Drawing for the job (mm, zero at the part's lowest x, y, z). A direction names the side the tool comes from. Round coordinates to 2 decimals unless told otherwise and drop trailing zeros. Loops run counter-clockwise (first coordinate to the right, second up) from the corner with the lowest first, then second, coordinate; pieces in that order, holes last. Notation, with made-up numbers: (-26.5, 26.25) -> (26.5, 26.25) arc R10 cw to (26.5, 41.25) -> close; hole circle Ø2 at (78.25, 80.25). An arc over 180 degrees is marked (long way). Put each result on its own line as item: value. Start each with the question number.
Item 1: Drill centre lines: probe 1 along Y at (x, z) = (55, 63); probe 2 along X at (y, z) = (133.5, 29.5); probe 3 along Y at (x, z) = (11, 50.5). Where is each one in solid material? Low to high. Write a range as [from, to].
Item 2: Cut at C-C, the plane z = 41. List the corners of the cut face in (x, y) (1 decimal).
Item 3: Tool access for the marked faces 1, 2, 3, 4 and 5: list every direction of +Z, -Z, +X, -X, +Y, -Y with a clear straight run to the whole face (end or side of a thin tool).
Item 4: Cut at B-B, the plane y = 129. List the corners of the cut face in (x, z) (1 decimal), plus the area to 3 significant figures.
Item 5: Cut at D-D, the plane x = 6. List the corners of the cut face in (y, z).
Item 6: Pull direction Y, two halves, no side cores. Call the marked faces 6, 7 and 8: +Y half, -Y half, draft (parallel to the pull), parting line (faces both ways), or undercut.
Item 7: Flat gauge pins, fed straight in: pin 1 Ø3 at (x, z) = (15.5, 47.5) entering from +Y; pin 2 Ø12 at (x, y) = (17.5, 152.5) entering from +Z; pin 3 Ø1.5 at (x, y) = (51.5, 293) entering from +Z (1 decimal); pin 4 Ø10 at (y, z) = (346.5, 50) entering from -X. Where does each tip first touch, or does it go through?
Item 8: Cut at A-A, the plane z = 23. List the corners of the cut face in (x, y) (1 decimal).
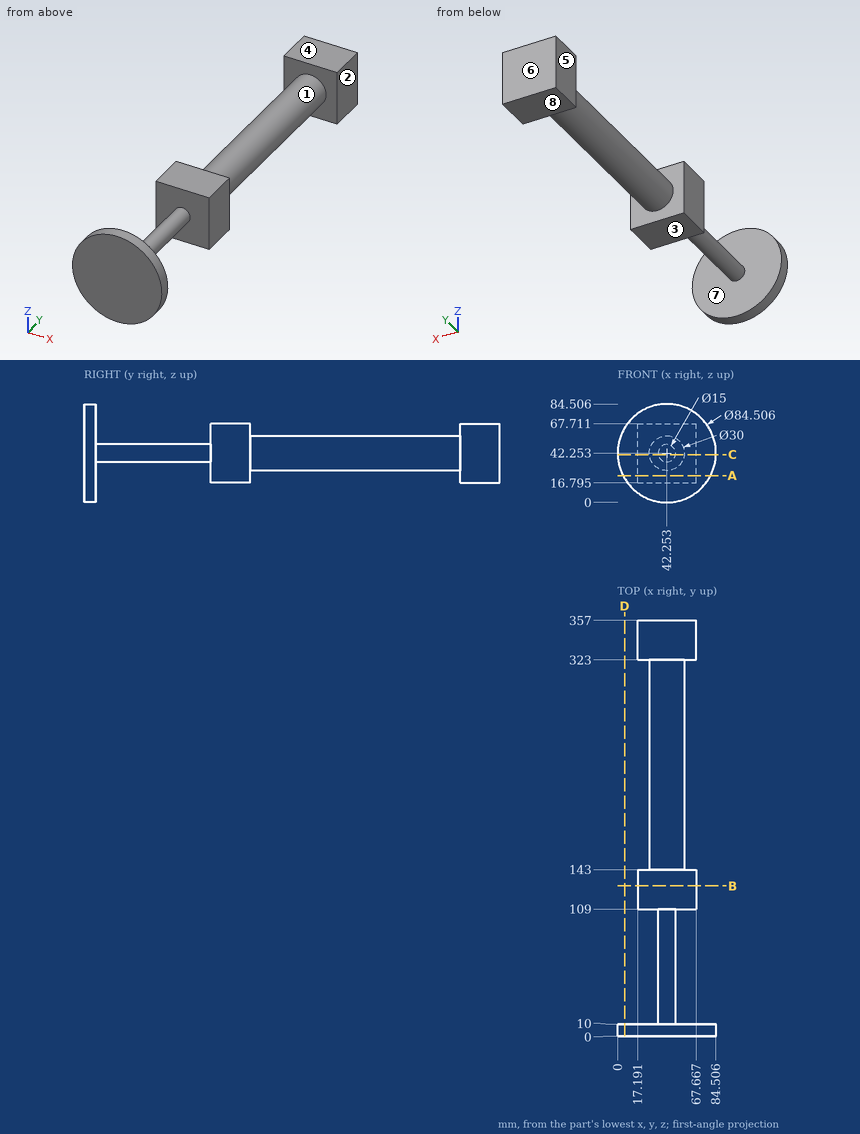
Reply:
1. probe 1: y = [0, 10], [109, 143], [323, 357]
1. probe 2: x = [17.19, 67.67]
1. probe 3: y = [0, 10]
2. outline: (0, 0) -> (84.5, 0) -> (84.5, 10) -> (49.6, 10) -> (49.6, 109) -> (67.7, 109) -> (67.7, 143) -> (57.2, 143) -> (57.2, 323) -> (67.7, 323) -> (67.7, 357) -> (17.2, 357) -> (17.2, 323) -> (27.3, 323) -> (27.3, 143) -> (17.2, 143) -> (17.2, 109) -> (34.9, 109) -> (34.9, 10) -> (0, 10) -> close
3. face 1: none
3. face 2: +Z, -Z, +X, +Y
3. face 3: -Z, +X, -X, +Y
3. face 4: +Z, +X, -X, +Y
3. face 5: +Z, -Z, -X, +Y
4. outline: (17.2, 16.8) -> (67.7, 16.8) -> (67.7, 67.7) -> (17.2, 67.7) -> close
4. area: 2,570 mm^2
5. outline: (0, 20.55) -> (10, 20.55) -> (10, 63.96) -> (0, 63.96) -> close
6. face 6: +Y half
6. face 7: undercut
6. face 8: draft
7. pin 1: stops at y = 10
7. pin 2: passes through
7. pin 3: stops at z = 54.6
7. pin 4: stops at x = 17.19
8. outline: (4.6, 0) -> (79.9, 0) -> (79.9, 10) -> (4.6, 10) -> close; (17.2, 109) -> (67.7, 109) -> (67.7, 143) -> (17.2, 143) -> close; (17.2, 323) -> (67.7, 323) -> (67.7, 357) -> (17.2, 357) -> close
